Geometry check sheet. Reference: the model listing, model coordinates, mm. A direction names the side the tool comes from. Coordinates: 2 decimals unless noted, no trailing zeros. Loops run counter-clockwise (first coordinate to the right, second up) from the corner with the lowest first, then second, coordinate; pieces in that order, holes last. Notation, with made-up numbers: (35, 66) -> (89, 66) arc R30 cw to (89, 93) -> close; hole circle Ø2 at (26, 4). An arc over 180 degrees is marked (long way). Answer as a JSON object with one key per item and string values.
from build123d import *

# Parameters (mm, degrees)
EXTRUDE_1_DEPTH     = 35
SKETCH_2_R          = 1.6
CUT_EXTRUDE_1_DEPTH = 43.234582986


with BuildPart() as part:
    # 草图1 → 凸台-拉伸1 (new body)
    with BuildSketch(Plane(origin=(0, 0, 0), x_dir=(1, 0, 0), z_dir=(0, 1, 0))):
        Polygon((0, 0), (0, 20), (12.6, 20), (12.6, 9.502030119), (12.6, 0), (11.9, 0), (11.9, 19.3), (0.7, 19.3), (0.7, 0), align=None)
    extrude(amount=EXTRUDE_1_DEPTH)

    # 草图2 → 切除-拉伸1 (cut, through all)
    with BuildSketch(Plane.ZY):
        with Locations((-5.2, 30.5)):
            Circle(SKETCH_2_R)
        with Locations((-5.2, 4.5)):
            Circle(SKETCH_2_R)
    extrude(amount=-CUT_EXTRUDE_1_DEPTH, mode=Mode.SUBTRACT)


solid = part.part
1. Depth check by flat-ended pin: P1, Ø3.5, axis at x = 4.5, y = 26, coming from the +Z side; P2, Ø1.5, axis at y = 25, z = -13, coming from the -X side. Enter the tip coordinate at first touch or a pass-through.
Evaluation:
{"P1": "stops at z = -19.3", "P2": "stops at x = 0"}
2. Section check A-A, the plane z = -5.2. Record the boundary of the cut face in (x, y), then the cut area to 3 significant figures.
Evaluation:
{"outline": "(0, 0) -> (0.7, 0) -> (0.7, 2.9) -> (0, 2.9) -> close; (0, 6.1) -> (0.7, 6.1) -> (0.7, 28.9) -> (0, 28.9) -> close; (0, 32.1) -> (0.7, 32.1) -> (0.7, 35) -> (0, 35) -> close; (11.9, 0) -> (12.6, 0) -> (12.6, 2.9) -> (11.9, 2.9) -> close; (11.9, 6.1) -> (12.6, 6.1) -> (12.6, 28.9) -> (11.9, 28.9) -> close; (11.9, 32.1) -> (12.6, 32.1) -> (12.6, 35) -> (11.9, 35) -> close", "area": "40.0 mm^2"}
3. Tool access check on faces 5 (the face through (0.345, 30.981, -3.674)), 6 (the face through (0.7, 17, -10)). Record the directions out of +Z, -Z, +X, -X, +Y, -Y that give a thin tool (end or side, any length) a straight path to the whole face; none if there is none.
Evaluation:
{"face 5": "+X, -X", "face 6": "+Z, +Y, -Y"}
4. Thickness scan on probe 1 along Y at (x, z) = (12.4, -5.2); probe 2 along X at (y, z) = (24, -14.75); probe 3 along Z at (x, y) = (7, 13.5). Record the ranges inside material, lowest first. Write a range as from..to.
Evaluation:
{"probe 1": "y = 0..2.9, 6.1..28.9, 32.1..35", "probe 2": "x = 0..0.7, 11.9..12.6", "probe 3": "z = -20..-19.3"}
5. Mould release check, pull along Y, two halves, no side actions. Record for faces 1 (the face through (0, 17, -10)), 2 (the face through (12.245, 30.981, -3.674)), 3 (the face through (12.4, 35, -12.3)), 4 (the face through (0.35, 3.89, -3.72)): released by +Y, released by -Y, zero draft, split by the parting line, or undercut.
Evaluation:
{"face 1": "zero draft", "face 2": "undercut", "face 3": "released by +Y", "face 4": "undercut"}
6. Section check B-B, the plane z = -1.5. Record the boundary of the cut face in (x, y), then the cut area to 3 significant figures.
Evaluation:
{"outline": "(0, 0) -> (0.7, 0) -> (0.7, 35) -> (0, 35) -> close; (11.9, 0) -> (12.6, 0) -> (12.6, 35) -> (11.9, 35) -> close", "area": "49.0 mm^2"}
7. Section check C-C, the plane y = 30.5. Record the boundary of the cut face in (x, z), then the cut area to 3 significant figures.
Evaluation:
{"outline": "(0, -20) -> (12.6, -20) -> (12.6, -6.8) -> (11.9, -6.8) -> (11.9, -19.3) -> (0.7, -19.3) -> (0.7, -6.8) -> (0, -6.8) -> close; (0, -3.6) -> (0.7, -3.6) -> (0.7, 0) -> (0, 0) -> close; (11.9, -3.6) -> (12.6, -3.6) -> (12.6, 0) -> (11.9, 0) -> close", "area": "31.4 mm^2"}
8. Section check D-D, the plane x = 9.5. Record the boundary of the cut face in (y, z).
Evaluation:
{"outline": "(0, -20) -> (35, -20) -> (35, -19.3) -> (0, -19.3) -> close"}
